from build123d import *

# Parameters (mm, degrees)
SKETCH2_W                  = 300
SKETCH2_H                  = 300
BOSS_EXTRUDE1_DEPTH        = 12
SKETCH3_R                  = 15
BOSS_EXTRUDE2_DEPTH        = 50
FILLET1_R                  = 7
F_12_0_12_DIAMETER_HOLE1_D = 12


with BuildPart() as part:
    # Sketch2 → Boss-Extrude1 (new body)
    with BuildSketch(Plane.XY):
        Rectangle(SKETCH2_W, SKETCH2_H)
    extrude(amount=BOSS_EXTRUDE1_DEPTH)

    # Sketch3 → Boss-Extrude2 (add)
    with BuildSketch(Plane.XY.offset(12)):
        with Locations((120, -120)):
            Circle(SKETCH3_R)
        with Locations((-120, -120)):
            Circle(SKETCH3_R)
        with Locations((-120, 120)):
            Circle(SKETCH3_R)
        with Locations((120, 120)):
            Circle(SKETCH3_R)
    extrude(amount=BOSS_EXTRUDE2_DEPTH)

    # Fillet1
    fillet1_edges = [part.edges().sort_by_distance(p)[0] for p in [
        (-135, -120, 62),
        (105, -120, 62),
        (-135, 120, 62),
        (105, 120, 62),
    ]]
    fillet(fillet1_edges, radius=FILLET1_R)

    # Ø12.0 (12) Diameter Hole1 (through all)
    with Locations(Plane.XY.offset(12)):
        with Locations((135, -90)):
            Hole(F_12_0_12_DIAMETER_HOLE1_D / 2)


solid = part.part
The model under review builds one solid part; all positions refer to its coordinate system, in mm. A direction names the side the tool comes from. Round coordinates to 2 decimals unless told otherwise and drop trailing zeros. Loops run counter-clockwise (first coordinate to the right, second up) from the corner with the lowest first, then second, coordinate; pieces in that order, holes last. Notation, with made-up numbers: (32, -14) -> (57, -14) arc R29 ccw to (57, 10) -> close; hole circle Ø2 at (54.25, 16.5). An arc over 180 degrees is marked (long way). One line per question, with ' | ' between items. Start each with the question number.
Item 1: For pin 1 (1 mm diameter, centred on x = 17.5, y = -70, fed in from +Z); pin 2 (19 mm diameter, centred on x = 135, y = -90, fed in from -Z), all flat-tipped, find the tip position at first contact; note any pin that passes through.
Item 2: Add section B-B, the plane z = 32. Write out the cut boundary in (x, y), then the cut area to 3 significant figures.
Item 3: Add section A-A, the plane y = -90. Write out the cut boundary in (x, z), then the cut area to 3 significant figures.
Item 4: Add section C-C, the plane x = -120. Write out the cut boundary in (y, z).
Item 5: Machinability: for faces 1 (the face through (-120, 120, 62)), 2 (the face through (-121.953, 134.872, 33.199)), which of the approach directions +Z, -Z, +X, -X, +Y, -Y give a long, thin tool a straight path to every point of the face, cutting with its end or side? Answer none if there is none.
Item 6: Draft analysis for pull direction Y (two halves, no side actions). For faces 3 (the face through (-2, 150, 6)), 4 (the face through (-120, -120, 62)), 5 (the face through (-131.056, -109.862, 33.199)), 6 (the face through (108.944, -109.862, 33.199)), state which applies: +Y half, -Y half, draft (parallel to the pull), parting line (faces both ways), or undercut.
Item 7: Wall thickness on line 1 along Y through (x, z) = (135, 5.25); line 2 along Z through (x, y) = (-4.5, -111); line 3 along Y through (x, z) = (131, 43.5): over which ranges is each line inside the solid? List them lowest first. Write a range as [from, to].
Return value:
1) pin 1: stops at z = 12 | pin 2: stops at z = 0
2) outline: circle Ø30 at (-120, -120); circle Ø30 at (-120, 120); circle Ø30 at (120, -120); circle Ø30 at (120, 120) | area: 2,830 mm2
3) outline: (-150, 0) -> (129, 0) -> (129, 12) -> (-150, 12) -> close; (141, 0) -> (150, 0) -> (150, 12) -> (141, 12) -> close | area: 3,460 mm2
4) outline: (-150, 0) -> (150, 0) -> (150, 12) -> (135, 12) -> (135, 55) arc R7 ccw to (128, 62) -> (112, 62) arc R7 ccw to (105, 55) -> (105, 12) -> (-105, 12) -> (-105, 55) arc R7 ccw to (-112, 62) -> (-128, 62) arc R7 ccw to (-135, 55) -> (-135, 12) -> (-150, 12) -> close
5) face 1: +Z, +X, -X, +Y, -Y | face 2: +Z
6) face 3: +Y half | face 4: draft | face 5: undercut | face 6: undercut
7) line 1: y = [-150, -96], [-84, 150] | line 2: z = [0, 12] | line 3: y = [-130.2, -109.8], [109.8, 130.2]
